The listing builds one solid part. Answer for the finished solid, in the listing's coordinates (mm). A direction names the side the tool comes from. Give positions to 0.01 mm unless a question says otherwise; leave off trailing zeros. Write each loop counter-clockwise with the first axis right and the second up, starting at its lowest first coordinate (ties: lowest second). Pieces come first, ordered by that corner, then holes. Notation, with made-up numbers: M -25.5,16.25 L 15.5,16.25 A32 cw 15.5,47.25 Z; hole C -16,7 d7. An arc over 180 degrees is marked long. Return JSON: item names as keys, results as strings.
Autodesk Inventor part; units mm, degrees
ref_plane "YZ Plane" through (0, 0, 0) normal (1, 0, 0) x (0, 1, 0)
ref_plane "XZ Plane" through (0, 0, 0) normal (0, 1, 0) x (-1, 0, 0)
ref_plane "XY Plane" through (0, 0, 0) normal (0, 0, 1) x (1, 0, 0)
sketch "Sketch1" plane through (0, 0, 0) normal (0, 1, 0) x (-1, 0, 0)
  line L0 (0, 0) -> (13.6144, 0)
  circle A0 centre (0, 0) radius 17.78
  dimension "d0" = 13.6144
  dimension "d1" = 35.56
extrude "Extrusion1" add sketch "Sketch1" along normal blind 19.05
sketch "Sketch3" plane through (0, 19.05, 0) normal (0, 1, 0) x (1, 0, 0)
  line L0 (0, 0) -> (0, 13.6144)
  line L1 (0, 0) -> (13.6144, 0) construction
  dimension "d4" = 13.6144
  dimension "d5" = 90
hole "Hole1" at (0, 19.05, -13.6144) direction (0, -1, 0) diameter 4.9022 end through all counterbore diameter 7.239 counterbore depth 5.08
sketch "Sketch4" plane through (0, 0, 0) normal (0, -1, 0) x (1, 0, 0)
  circle A0 centre (0, -13.6144) radius 2.4511
  line L0 (0, 0) -> (0, -13.6144)
hole "Hole2" at (0, 0, -13.6144) direction (0, 1, 0) diameter 4.9022 depth 6.35
pattern_circular "Circular Pattern1" count 3 over 360 about axis through (0, 0, 0) along (0, 1, 0) of "Hole1", "Hole2"
sketch "Sketch6" plane through (0, 19.05, 0) normal (0, 1, 0) x (1, 0, 0)
  point P0 (0, 0)
  point P1 (0, 0)
hole "Hole3" at (0, 19.05, 0) direction (0, -1, 0) diameter 6.35 end through all
sketch "Sketch14" plane through (0, 0, 0) normal (0, -1, 0) x (1, 0, 0)
  circle A0 centre (11.7904, 6.8072) radius 2.4511
  circle A1 centre (0, -13.6144) radius 2.4511
  circle A2 centre (-11.7904, 6.8072) radius 2.4511
  line L0 (11.7904, 6.8072) -> (0, 0)
  line L1 (0, 0) -> (11.7904, 6.8072)
  line L2 (-11.7904, 6.8072) -> (0, -13.6144)
  line L3 (0, -13.6144) -> (11.7904, 6.8072)
  line L4 (-11.7904, 6.8072) -> (11.7904, 6.8072)
  line L5 (-11.7904, 6.8072) -> (5.8952, -3.4036)
  line L6 (0, -13.6144) -> (0, 6.8072)
  line L7 (11.7904, 6.8072) -> (-5.8952, -3.4036)
  circle A3 centre (11.7904, 6.8072) radius 2.4511
  line L8 (13.9131, 8.0328) -> (15.3979, 8.89)
  circle A4 centre (0, 0) radius 17.78
  circle A5 centre (0, 0) radius 16.0655
properties part number "tablebackup"
Item 1: Find the intervals of material crossed by line 1 (X direction, y = 17.75, z = 6.5); line 2 (Z direction, x = -0.5, y = 9.25); line 3 (X direction, y = 6.75, z = 5), in increasing order.
Geometry results:
{"line 1": "x = -16.55 to -15.4, -8.18 to 8.18, 15.4 to 16.55", "line 2": "z = -17.77 to -16.01, -11.21 to -3.14, 3.14 to 17.77", "line 3": "x = -17.06 to -13.45, -10.13 to 10.13, 13.45 to 17.06"}
Item 2: Which of the six approach directions +Z, -Z, +X, -X, +Y, -Y give full straight-line access (tool end or side, diameter ignored) to faces 4 (the flat face through (9, 13.97, 6)), 5 (the cylindrical face through (-10.3, 6.89, 4.86))?
Geometry results:
{"face 4": "+Y", "face 5": "+Y, -Y"}
Item 3: A cutting plane is placed at A-A, the plane z = 0. Write down the section's boundary in (x, y) (3 decimals).
Geometry results:
{"outline": "M -17.78,0 L -3.175,0 L -3.175,19.05 L -17.78,19.05 Z; M 3.175,0 L 17.78,0 L 17.78,19.05 L 3.175,19.05 Z"}
Item 4: A cutting plane is placed at D-D, the plane x = -13. Write down the section's boundary in (y, z), plus the area to 3 significant figures.
Geometry results:
{"outline": "M 0,-12.13 L 19.05,-12.13 L 19.05,3.4 L 13.97,3.4 L 13.97,4.68 L 0,4.68 Z; M 0,8.94 L 13.97,8.94 L 13.97,10.22 L 19.05,10.22 L 19.05,12.13 L 0,12.13 Z", "area": "368 mm2"}
Item 5: A cutting plane is placed at B-B, the plane x = 0. Count the separate pieces of the cut face and the enclosed holes in it, plus the area to 3 significant figures.
Geometry results:
{"separate pieces": "3", "enclosed holes": "0", "area": "451 mm2"}
Item 6: Determine the mould class of faces 1 (the cylindrical face through (3.85, 9.39, 17.36)), 2 (the cylindrical face through (3.1, 9.39, -0.69)), 3 (the flat face through (-4, 0, 0)) for opening direction Z: +Z half, -Z half, draft (parallel to the pull), parting line (faces both ways), or undercut.
Geometry results:
{"face 1": "parting line", "face 2": "undercut", "face 3": "draft"}
Item 7: A cutting plane is placed at C-C, the plane y = 11.75. Write down the section's boundary in (x, z) (3 decimals), plus the area to 3 significant figures.
Geometry results:
{"outline": "C 0,0 d35.56; hole C -11.79,6.807 d4.902; hole C 0,0 d6.35; hole C 0,-13.614 d4.902; hole C 11.79,6.807 d4.902", "area": "905 mm2"}
Item 8: Given pin 1 Ø6.5 at (x, z) = (0, -13.61) entering from +Y; pin 2 Ø5 at (x, y) = (-5, 8) entering from -Z; pin 3 Ø4 at (x, z) = (11.79, 6.81) entering from -Y; pin 4 Ø5 at (y, z) = (7.5, 8) entering from +X, each flat-ended and moving along its own axis, determine where each tip first touches the part or whether it passes through.
Geometry results:
{"pin 1": "stops at y = 13.97", "pin 2": "stops at z = -17.6", "pin 3": "passes through", "pin 4": "stops at x = 16.91"}
